Design review of the part shown in the three views and the two pictorial views. Dimensions are in mm from the part's minimum x, y and z. Give positions to 0.01 mm unless a question says otherwise; leave off trailing zeros. Order: outer loops, then holes, each group sorted by start corner. A loop starts at its lowest first (then second) coordinate and runs counter-clockwise, first axis right, second up.
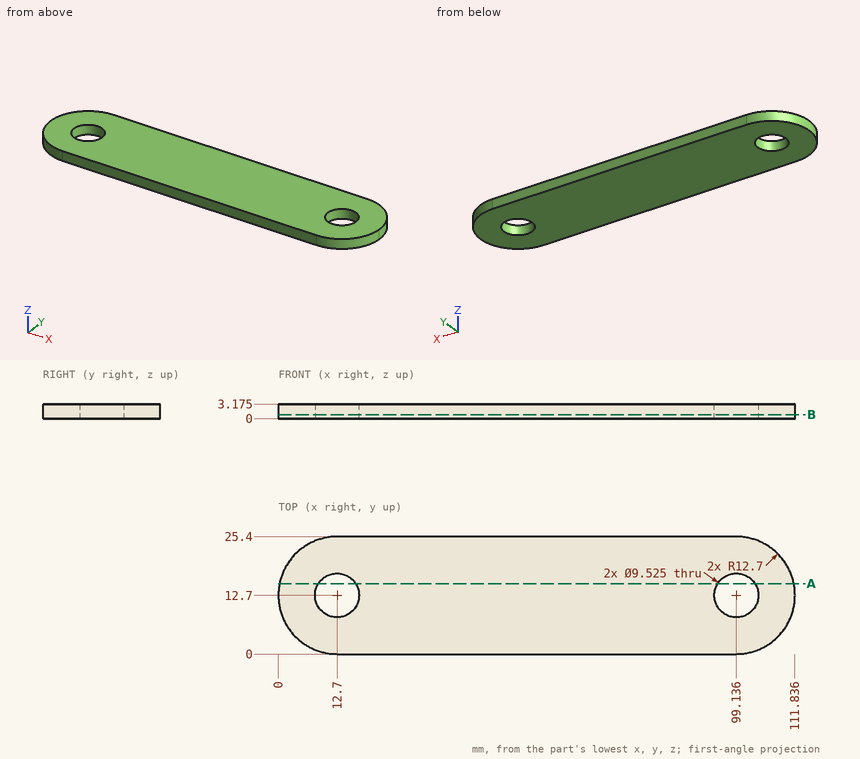
1) To check wall thickness, follow line 1 (X direction, y = 12.5, z = 1.55) (1 decimal); line 2 (X direction, y = 11.25, z = 1.75); line 3 (Y direction, x = 9, z = 1.3). State the ranges of each line that lie inside material, in increasing order.
Answer sheet:
line 1: x = 0 to 7.9, 17.5 to 94.4, 103.9 to 111.8
line 2: x = 0.08 to 8.16, 17.24 to 94.6, 103.67 to 111.75
line 3: y = 0.55 to 9.7, 15.7 to 24.85
2) We need section B-B on z = 0.9. Give the boundary of the cut face in (x, y) (1 decimal).
Answer sheet:
outline: (12.7, 0) - (99.1, 0) arc R12.7 ccw to (99.1, 25.4) - (12.7, 25.4) arc R12.7 ccw to start; hole circle Ø9.5 at (12.7, 12.7); hole circle Ø9.5 at (99.1, 12.7)
3) We need section A-A on y = 15.25. Give the boundary of the cut face in (x, z) (1 decimal), then the cut area to 3 significant figures.
Answer sheet:
outline: (0.3, 0) - (8.7, 0) - (8.7, 3.2) - (0.3, 3.2) - close; (16.7, 0) - (95.1, 0) - (95.1, 3.2) - (16.7, 3.2) - close; (103.2, 0) - (111.6, 0) - (111.6, 3.2) - (103.2, 3.2) - close
area: 302 mm2
4) Clearance check with flat-ended pins moving along their axes: pin 1 (2 mm diameter, centred on x = 94.5, y = 12.5, fed in from -Z); pin 2 (1.5 mm diameter, centred on y = 8.5, z = 1.5, fed in from +X). State where each tip first meets the part, or that it passes through.
Answer sheet:
pin 1: stops at z = 0
pin 2: stops at x = 111.36
